CAD build for the part. Positions are in the model's coordinates, mm. A direction names the side the tool comes from. Round coordinates to 2 decimals unless told otherwise and drop trailing zeros. Order: outer loops, then holes, each group sorted by start corner. A loop starts at its lowest first (then second) coordinate and runs counter-clockwise, first axis right, second up. Notation, with made-up numbers: (-2.75, -3) -> (31.25, -3) arc R16 ccw to (31.25, 14) -> close; hole circle Ø1 at (27, 69). An arc over 180 degrees is marked (long way). Return JSON: item names as keys, results as strings. Group by question number.
Q1. Cut at A-A (y = -44). Write the cut outline in (x, z), then the cut area to 3 significant figures.
Q2. Flat gauge pins, fed straight in: pin 1 (1 mm diameter, centred on x = -4.5, y = 37, fed in from -Z); pin 2 (5.5 mm diameter, centred on x = 24.5, y = -44, fed in from -Z); pin 3 (4.5 mm diameter, centred on x = 24.5, y = 14, fed in from -Z); pin 4 (3 mm diameter, centred on x = -24.5, y = -44, fed in from +Z). Where does each tip first touch, or does it go through?
Q3. Probe line 1 along Y through (x, z) = (24.5, 2.55); line 2 along Y through (x, z) = (27, 1.9); line 3 along X through (y, z) = (-44.5, 1.4). List the from-to ranges inside material, lowest first.
Q4. Cut at B-B (x = -24.5). Write the cut outline in (y, z), then the cut area to 3 significant figures.
Q5. Mould opens along X. For faces 1 (the flat face through (-32.5, 1, 1)), 2 (the flat face through (20, 51, 1)), 3 (the flat face through (0, 2, 0)), 4 (the cylindrical face through (-24.88, -45.71, 2.51)) say: +X half, -X half, draft (parallel to the pull), parting line (faces both ways), or undercut.
Q6. Cut at C-C (z = 1). Write the cut outline in (x, y), then the cut area to 3 significant figures.
Q7. Which spindle directions (+Z, -Z, +X, -X, +Y, -Y) get a long thin tool onto all of the face, cutting with end or side? Do faces 5 (the flat face through (-20, 51, 1)), 6 (the flat face through (26, 50, 1)), 7 (the cylindrical face through (-25.79, 15.18, 2.51)). Say none if no direction does.
from build123d import *

# Parameters (mm, degrees)
SKETCH_1_W          = 40
SKETCH_1_H          = 3
EXTRUDE_1_DEPTH     = 3
SKETCH_2_R          = 1.75
CUT_EXTRUDE_1_DEPTH = 10
CHAMFER_1_SIZE      = 2


with BuildPart() as part:
    # Эскиз1 → Бобышка-Вытянуть1 (new body)
    with BuildSketch(Plane.XY):
        Polygon((-32.5, 50), (-32.5, -50), (32.5, -50), (32.5, 50), (20, 50), (20, 47), (-20, 47), (-20, 50), align=None)
        with Locations((0, 48.5)):
            Rectangle(SKETCH_1_W, SKETCH_1_H)
        with Locations((0, 51.5)):
            Rectangle(SKETCH_1_W, SKETCH_1_H)
    extrude(amount=EXTRUDE_1_DEPTH)

    # Эскиз2 → Вырез-Вытянуть1 (cut)
    with BuildSketch(Plane.XY.offset(3)):
        with Locations((-24.5, 14)):
            Circle(SKETCH_2_R)
        with Locations((24.5, 14)):
            Circle(SKETCH_2_R)
        with Locations((24.5, -44)):
            Circle(SKETCH_2_R)
        with Locations((-24.5, -44)):
            Circle(SKETCH_2_R)
    extrude(amount=-CUT_EXTRUDE_1_DEPTH, mode=Mode.SUBTRACT)

    # Фаска1
    chamfer_1_edges = [part.edges().sort_by_distance(p)[0] for p in [
        (-26.25, -44, 0),
        (22.75, -44, 0),
        (22.75, 14, 0),
        (-26.25, 14, 0),
    ]]
    chamfer(chamfer_1_edges, length=CHAMFER_1_SIZE)


solid = part.part
Solution:
{
 "1": {"outline": "(-32.5, 0) -> (-28.25, 0) -> (-26.25, 2) -> (-26.25, 3) -> (-32.5, 3) -> close; (-22.75, 2) -> (-20.75, 0) -> (20.75, 0) -> (22.75, 2) -> (22.75, 3) -> (-22.75, 3) -> close; (26.25, 2) -> (28.25, 0) -> (32.5, 0) -> (32.5, 3) -> (26.25, 3) -> close", "area": "166 mm²"},
 "2": {"pin 1": "stops at z = 0", "pin 2": "stops at z = 1", "pin 3": "stops at z = 1.5", "pin 4": "passes through"},
 "3": {"line 1": "y = -50 to -45.75, -42.25 to 12.25, 15.75 to 50", "line 2": "y = -50 to 50", "line 3": "x = -32.5 to -26.8, -22.2 to 22.2, 26.8 to 32.5"},
 "4": {"outline": "(-50, 0) -> (-47.75, 0) -> (-45.75, 2) -> (-45.75, 3) -> (-50, 3) -> close; (-42.25, 2) -> (-40.25, 0) -> (10.25, 0) -> (12.25, 2) -> (12.25, 3) -> (-42.25, 3) -> close; (15.75, 2) -> (17.75, 0) -> (50, 0) -> (50, 3) -> (15.75, 3) -> close", "area": "271 mm²"},
 "5": {"face 1": "-X half", "face 2": "+X half", "face 3": "draft", "face 4": "undercut"},
 "6": {"outline": "(-32.5, -50) -> (32.5, -50) -> (32.5, 50) -> (20, 50) -> (20, 53) -> (-20, 53) -> (-20, 50) -> (-32.5, 50) -> close; hole circle Ø5.5 at (-24.5, -44); hole circle Ø5.5 at (-24.5, 14); hole circle Ø5.5 at (24.5, -44); hole circle Ø5.5 at (24.5, 14)", "area": "6,520 mm²"},
 "7": {"face 5": "+Z, -Z, -X, +Y", "face 6": "+Z, -Z, +X, +Y", "face 7": "+Z, -Z"}
}
